```python
from build123d import *

# Parameters (mm, degrees)
F2_W     = 76.4627605677
F2_H     = 78.6305181682
F3_DEPTH = 35.561
F4_SIZE  = 1.27
F6_D     = 4.953
F6_DEPTH = 11.43
F6_TIP   = 1.488031323


with BuildPart() as f1:
    # F0 (on Front) → F1 (revolve)
    with BuildSketch(Plane.XZ):
        Polygon((-49.911, 11.43), (0, 11.43), (0, 13.4529743879), (-0.8980256121, 14.351), (-15.1220256121, 14.351), (-16.7095256121, 17.100630657), (-32.258, 17.100630657), (-32.258, 22.479), (-49.53, 22.479), (-49.53, 28.7401), (-62.103, 28.7401), (-62.103, 35.56), (-66.294, 35.56), (-66.294, 20.0533), (-69.596, 20.0533), (-69.596, 11.43), (-55.626, 11.43), (-55.626, 13.843), (-49.911, 13.843), align=None)
    revolve(axis=Axis((-34.5281772316, 0, 0), (-1, 0, 0)))

    # F2 (on Front) → F3 (cut, through all)
    with BuildSketch(Plane.XZ):
        with Locations((-38.2313802838, 0.098535791)):
            Rectangle(F2_W, F2_H)
    extrude(amount=F3_DEPTH, mode=Mode.SUBTRACT)

    # F4
    f4_edges = [f1.edges().sort_by_distance(p)[0] for p in [
        (-69.596, 20.0533, 0),
        (-49.53, 28.7401, 0),
        (-32.258, 22.479, 0),
    ]]
    chamfer(f4_edges, length=F4_SIZE)

    # F6
    with Locations(Plane(origin=(-69.596, 0, 0), x_dir=(0, -1, 0), z_dir=(-1, 0, 0))):
        with Locations((-14.1731563031, 0)):
            Hole(F6_D / 2, depth=F6_DEPTH)
            with Locations((0, 0, -(F6_DEPTH + F6_TIP / 2))):  # 118° drill point
                Cone(0, F6_D / 2, F6_TIP, mode=Mode.SUBTRACT)


solid = f1.part
```
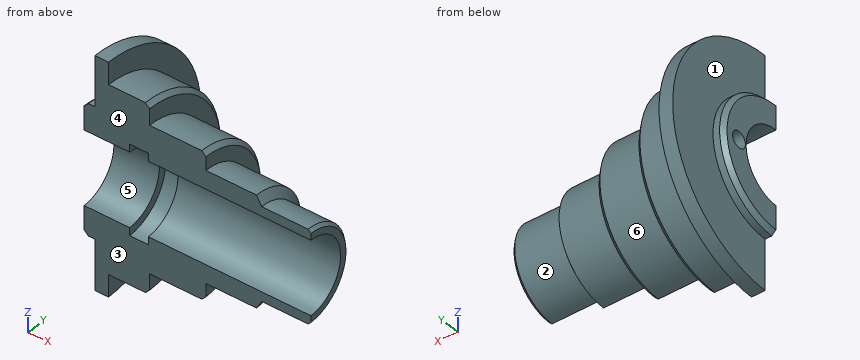
Work out the finished part from the listing and answer in its coordinate system (mm). Face numbers are marked on the shaded views. A direction names the side the tool comes from. Round coordinates to 2 decimals unless told otherwise and drop trailing zeros. Write each loop counter-clockwise with the first axis right and the second up, starting at its lowest first coordinate (ties: lowest second). Pieces come first, ordered by that corner, then holes. Notation, with made-up numbers: (-9.75, 89.5) - (20.25, 89.5) arc R34 cw to (20.25, 119.5) - close; hole circle Ø7 at (67, -38.5). An arc over 180 degrees is marked (long way). Return JSON: item names as keys, results as strings. Group by question number.
Q1. The part is cut by section A-A on x = -54.5. Write down the section's boundary in (y, z), then the cut area to 3 significant figures.
Q2. Each of these flat-tipped pins is pushed along its axis until it touches: pin 1 Ø2 at (x, y) = (-43.5, 10.5) entering from -Z; pin 2 Ø4 at (x, y) = (-48.5, 12) entering from +Z; pin 3 Ø6 at (x, y) = (-51, 26.5) entering from +Z. Where does it stop, or does it pass through?
Q3. For the marked faces 1, 2 and 3, determine the directions among +Z, -Z, +X, -X, +Y, -Y from which every point of the face is accessible in a straight line to the end or side of a thin tool.
Q4. The mould has two halves that part along Z. Classify the marked faces 4, 5 and 6: released by +Z, released by -Z, zero draft, split by the parting line, or undercut.
Q5. Find the intervals of material crossed by L1, parallel to Y at x = -66.25, z = 0; L2, parallel to Y at x = -61, z = 0; L3, parallel to X at y = 23.5, z = -9, in increasing order.
Q6. The part is cut by section B-B on x = -42.5. Write down the section's boundary in (y, z), then the cut area to 3 significant figures.
Solved:
{
 "1": {"outline": "(0, -28.74) arc R28.74 ccw to (0, 28.74) - (0, 13.84) arc R13.84 cw to (0, -13.84) - close", "area": "996 mm²"},
 "2": {"pin 1": "z = -20.37", "pin 2": "z = 25.96", "pin 3": "z = 16.55"},
 "3": {"face 1": "-X, +Y", "face 2": "+X, +Y", "face 3": "+Z, -Z, +X, -X, -Y"},
 "4": {"face 4": "zero draft", "face 5": "undercut", "face 6": "split by the parting line"},
 "5": {"L1": "11.43 to 11.7, 16.65 to 35.56", "L2": "11.43 to 11.7, 16.65 to 28.74", "L3": "-66.29 to -49.53"},
 "6": {"outline": "(0, -22.48) arc R22.48 ccw to (0, 22.48) - (0, 11.43) arc R11.43 cw to (0, -11.43) - close", "area": "589 mm²"}
}
